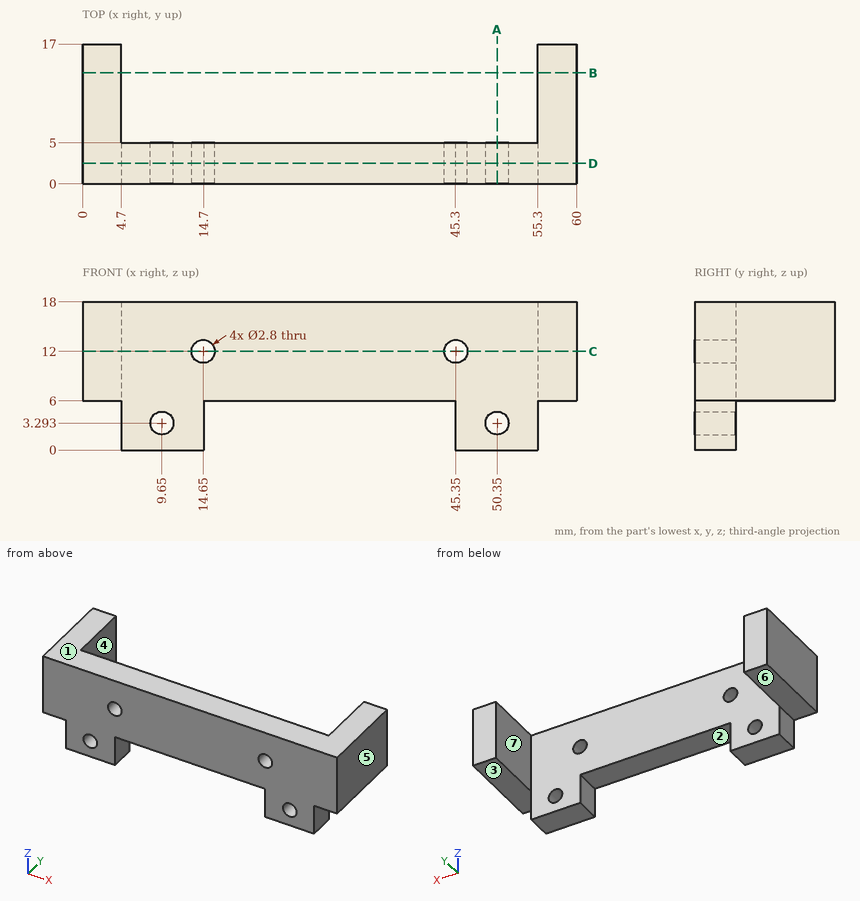
Verification items for this drawing (mm, ordinates from the low corner). A direction names the side the tool comes from. Round coordinates to 2 decimals unless told otherwise and drop trailing zeros. Order: outer loops, then holes, each group sorted by start corner. A loop starts at its lowest first (then second) coordinate and runs counter-clockwise, first axis right, second up.
1) Cross-section at C-C, the plane z = 12. Record the cut outline in (x, y).
Geometry says:
outline: (0, 0) - (13.25, 0) - (13.25, 5) - (4.7, 5) - (4.7, 17) - (0, 17) - close; (16.05, 0) - (43.95, 0) - (43.95, 5) - (16.05, 5) - close; (46.75, 0) - (60, 0) - (60, 17) - (55.3, 17) - (55.3, 5) - (46.75, 5) - close
2) Material ranges on line 1 (X direction, y = 1.55, z = 12); line 2 (X direction, y = 15.5, z = 13.75); line 3 (Z direction, x = 14.65, y = 2.1), recorded low to high.
Geometry says:
line 1: x = 0 to 13.25, 16.05 to 43.95, 46.75 to 60
line 2: x = 0 to 4.7, 55.3 to 60
line 3: z = 0 to 10.6, 13.4 to 18
3) Cross-section at D-D, the plane y = 2.5. Record the cut outline in (x, z).
Geometry says:
outline: (0, 6) - (4.7, 6) - (4.7, 0) - (14.7, 0) - (14.7, 6) - (45.3, 6) - (45.3, 0) - (55.3, 0) - (55.3, 6) - (60, 6) - (60, 18) - (0, 18) - close; hole circle Ø2.8 at (9.65, 3.29); hole circle Ø2.8 at (14.65, 12); hole circle Ø2.8 at (45.35, 12); hole circle Ø2.8 at (50.35, 3.29)
4) Cross-section at B-B, the plane y = 13.5. Record the cut outline in (x, z).
Geometry says:
outline: (0, 6) - (4.7, 6) - (4.7, 18) - (0, 18) - close; (55.3, 6) - (60, 6) - (60, 18) - (55.3, 18) - close
5) Draft check along X on the marked faces 5, 6 and 7. Enter one of: +X half, -X half, draft (parallel to the pull), parting line (faces both ways), or undercut.
Geometry says:
face 5: +X half
face 6: draft
face 7: undercut
6) Cross-section at A-A, the plane x = 50.35. Record the cut outline in (y, z), plus the area to 3 significant figures.
Geometry says:
outline: (0, 0) - (5, 0) - (5, 1.89) - (0, 1.89) - close; (0, 4.69) - (5, 4.69) - (5, 18) - (0, 18) - close
area: 76.0 mm2
7) Depth check by flat-ended pin: pin 1 (4 mm diameter, centred on x = 57, y = 7, fed in from -Z); pin 2 (10 mm diameter, centred on x = 13.5, z = 4.5, fed in from +Y); pin 3 (1.5 mm diameter, centred on y = 3.5, z = 3, fed in from -X). Enter the tip coordinate at first touch or a pass-through.
Geometry says:
pin 1: stops at z = 6
pin 2: stops at y = 5
pin 3: stops at x = 4.7
8) Tool access check on the marked faces 1, 2, 3 and 4. Record the directions out of +Z, -Z, +X, -X, +Y, -Y that give a thin tool (end or side, any length) a straight path to the whole face; none if there is none.
Geometry says:
face 1: +Z, +X, -X, +Y, -Y
face 2: -Z, +Y, -Y
face 3: -Z, +X, +Y, -Y
face 4: +Z, -Z, +Y
